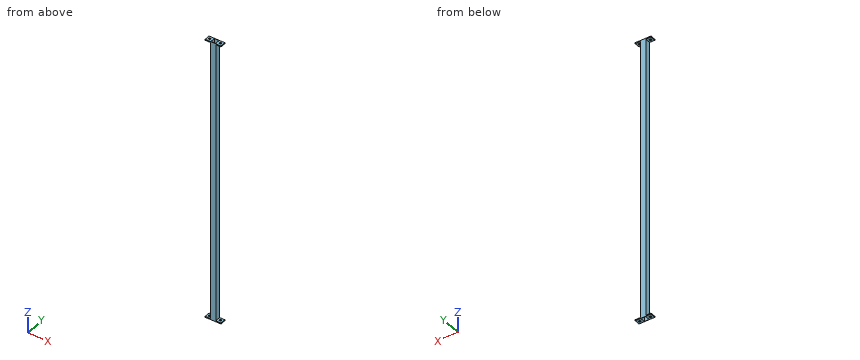
Autodesk Inventor part; units mm, degrees
ref_plane "YZ Plane" through (0, 0, 0) normal (1, 0, 0) x (0, 1, 0)
ref_plane "XZ Plane" through (0, 0, 0) normal (0, 1, 0) x (-1, 0, 0)
ref_plane "XY Plane" through (0, 0, 0) normal (0, 0, 1) x (1, 0, 0)
sketch "Sketch2" plane through (0, 0, 0) normal (0, 0, 1) x (1, 0, 0)
  line L0 (0, 0) -> (31.75, 0)
  line L1 (31.75, 0) -> (31.75, 31.75)
  line L2 (31.75, 31.75) -> (0, 31.75)
  line L3 (0, 31.75) -> (0, 0)
  line L4 (2, 29.75) -> (29.75, 29.75)
  line L5 (29.75, 29.75) -> (29.75, 2)
  line L6 (29.75, 2) -> (2, 2)
  line L7 (2, 2) -> (2, 29.75)
  dimension "d0" = 31.75
  dimension "d1" = 31.75
  dimension "d2" = 2
extrude "Extrusion1" add sketch "Sketch2" along normal blind 1650
sketch "Sketch3" plane through (0, 0, 1650) normal (0, 0, 1) x (1, 0, 0)
  line L0 (31.75, 31.75) -> (0, 31.75)
  line L1 (0, 31.75) -> (-30, 31.75)
  line L2 (-30, 31.75) -> (-30, 0)
  line L3 (-30, 0) -> (0, 0)
  line L4 (0, 0) -> (0, 31.75)
  line L5 (31.75, 31.75) -> (61.75, 31.75)
  line L6 (61.75, 31.75) -> (61.75, 0)
  line L7 (61.75, 0) -> (31.75, 0)
  line L8 (31.75, 0) -> (31.75, 31.75)
  circle A0 centre (-15, 15.875) radius 6
  circle A1 centre (46.75, 15.875) radius 6
  dimension "d5" = 30
  dimension "d6" = 30
  dimension "d7" = 12
  dimension "d8" = 12
extrude "Extrusion2" add sketch "Sketch3" against normal blind 6
sketch "Sketch4" plane through (0, 0, 0) normal (0, 0, -1) x (-1, 0, 0)
  line L0 (-61.75, 31.75) -> (30, 31.75)
  line L1 (30, 0) -> (-61.75, 0)
  line L2 (0, 31.75) -> (30, 31.75)
  line L3 (30, 31.75) -> (30, 0)
  line L4 (30, 0) -> (0, 0)
  line L5 (0, 0) -> (0, 31.75)
  line L6 (-31.75, 31.75) -> (-31.75, 0)
  line L7 (-31.75, 31.75) -> (-61.75, 31.75)
  line L8 (-61.75, 31.75) -> (-61.75, 0)
  line L9 (-61.75, 0) -> (-31.75, 0)
  line L10 (-31.75, 0) -> (-31.75, 31.75)
  circle A0 centre (-46.75, 15.875) radius 6
  circle A1 centre (-46.75, 15.875) radius 6
  circle A2 centre (15, 15.875) radius 6
  dimension "d11" = 30
  dimension "d12" = 12
extrude "Extrusion3" add sketch "Sketch4" against normal blind 6 contours L0 L6 L1 L8 | L0 L3 L1 L5
properties part number "Bases_Perfiles_Acero"
Input: part model. Units: mm. Frame: model coordinates. Round coordinates to 2 decimals unless told otherwise and drop trailing zeros. Loops run counter-clockwise (first coordinate to the right, second up) from the corner with the lowest first, then second, coordinate; pieces in that order, holes last. Notation, with made-up numbers: M 66,48.25 L 81,48.25 A11 cw 81,64.25 Z; hole C 45.25,24 d6. An arc over 180 degrees is marked long. Answer in a Markdown table with one row per item. Add a question column.
1. Section A-A (z = 1146). Output: boundary loops of the cut face in (x, y).
2. Ray query, probe 1 along X at (y, z) = (26.5, 1113.5); probe 2 along Z at (x, y) = (57.5, 15.5). Return the intervals inside material, ascending.
3. Contact query for flat-ended pins moving along their axis: pin 1 (14 mm diameter, centred on y = 21, z = 979, fed in from +X); pin 2 (9.5 mm diameter, centred on x = -15, y = 15.875, fed in from -Z); pin 3 (1.5 mm diameter, centred on y = 4, z = 283.5, fed in from -X). Output: stop coordinate, or through.
Values follow:
| question | item | result |
|---|---|---|
| 1 | outline | M 0,0 L 31.75,0 L 31.75,31.75 L 0,31.75 Z; hole M 2,2 L 29.75,2 L 29.75,29.75 L 2,29.75 Z |
| 2 | probe 1 | 0 to 2, 29.75 to 31.75 |
| 2 | probe 2 | 0 to 6, 1644 to 1650 |
| 3 | pin 1 | x = 31.75 |
| 3 | pin 2 | through |
| 3 | pin 3 | x = 0 |
